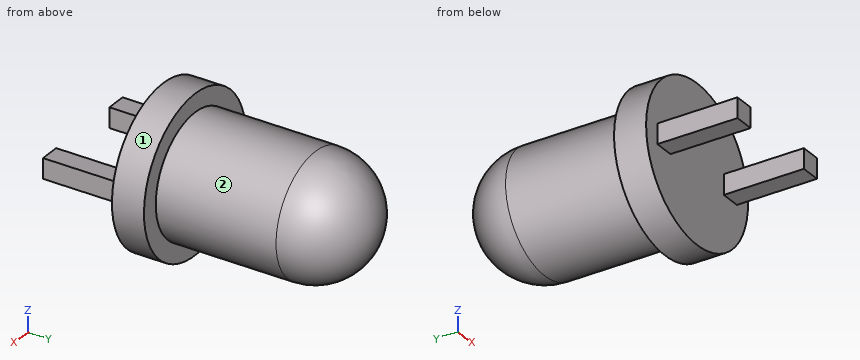
from build123d import *

# Parameters (mm, degrees)
SKETCH_1_W      = 1.95
SKETCH_1_H      = 0.8
SKETCH_2_W      = 0.5
SKETCH_2_H      = 0.5
EXTRUDE_1_DEPTH = 2


with BuildPart() as part:
    # Эскиз1 → Повернуть1 (revolve)
    with BuildSketch(Plane.XY, mode=Mode.PRIVATE) as revolve_1_sk:
        with BuildLine():
            Line((-1.5, 0.8), (0, 0.8))
            Line((0, 0.8), (0, 5.3))
            ThreePointArc((0, 5.3), (-1.060660172, 4.860660172), (-1.5, 3.8))
            Line((-1.5, 3.8), (-1.5, 0.8))
        make_face()
        with Locations((-0.975, 0.4)):
            Rectangle(SKETCH_1_W, SKETCH_1_H)
    revolve(revolve_1_sk.sketch.rotate(Axis((0, 8.783857323, 0), (0, -1, 0)), 270), axis=Axis((0, 8.783857323, 0), (0, -1, 0)))

    # Эскиз2 → Бобышка-Вытянуть1 (add)
    with BuildSketch(Plane.XZ):
        with Locations((-1.27, 0)):
            Rectangle(SKETCH_2_W, SKETCH_2_H)
        with Locations((1.27, 0)):
            Rectangle(SKETCH_2_W, SKETCH_2_H)
    extrude(amount=EXTRUDE_1_DEPTH)


solid = part.part
The model under review builds one solid part; all positions refer to its coordinate system, in mm. Face numbers are marked on the shaded views. A direction names the side the tool comes from. Coordinates: 2 decimals unless noted, no trailing zeros. Write each loop counter-clockwise with the first axis right and the second up, starting at its lowest first coordinate (ties: lowest second). Pieces come first, ordered by that corner, then holes. Notation, with made-up numbers: (14, -6.75) -> (31, -6.75) arc R14 cw to (31, 0.25) -> close; hole circle Ø2 at (47.25, 66). An arc over 180 degrees is marked (long way). Answer in a Markdown table with one row per item.
1. Wall thickness on probe 1 along X at (y, z) = (-0.5, -0.1); probe 2 along X at (y, z) = (4.5, 0.85); probe 3 along Y at (x, z) = (0.1, -1.7): over which ranges is each line inside the solid? List them lowest first. Write a range as [from, to].
Answers below:
| item | result |
|---|---|
| probe 1 | x = [-1.52, -1.02], [1.02, 1.52] |
| probe 2 | x = [-1.02, 1.02] |
| probe 3 | y = [0, 0.8] |
2. For the marked faces 1 and 2, list the 3-axis set-ups (+Z, -Z, +X, -X, +Y, -Y) from which the entire face can be reached by the end or side of a thin tool; tool diameter is ignored.
Answers below:
| item | result |
|---|---|
| face 1 | +Y, -Y |
| face 2 | +Y |
3. We need section D-D, the plane y = 1.5. State the section outline as (x, z) points, and give its area (3 significant figures).
Answers below:
| item | result |
|---|---|
| outline | circle Ø3 at (0, 0) |
| area | 7.07 mm^2 |
4. Clearance check with flat-ended pins moving along their axes: pin 1 Ø0.6 at (x, y) = (-1.5, -1) entering from -Z; pin 2 Ø0.6 at (y, z) = (-1, 0) entering from -X; pin 3 Ø0.6 at (x, y) = (1.5, -1) entering from +Z. State where each tip first meets the part, or that it passes through.
Answers below:
| item | result |
|---|---|
| pin 1 | stops at z = -0.25 |
| pin 2 | stops at x = -1.52 |
| pin 3 | stops at z = 0.25 |
5. We need section A-A, the plane y = -1. State the section outline as (x, z) points.
Answers below:
| item | result |
|---|---|
| outline | (-1.52, -0.25) -> (-1.02, -0.25) -> (-1.02, 0.25) -> (-1.52, 0.25) -> close; (1.02, -0.25) -> (1.52, -0.25) -> (1.52, 0.25) -> (1.02, 0.25) -> close |
6. We need section B-B, the plane x = 0. State the section outline as (y, z) points.
Answers below:
| item | result |
|---|---|
| outline | (0, -1.95) -> (0.8, -1.95) -> (0.8, -1.5) -> (3.8, -1.5) arc R1.5 ccw to (3.8, 1.5) -> (0.8, 1.5) -> (0.8, 1.95) -> (0, 1.95) -> close |
7. We need section C-C, the plane z = 0. State the section outline as (x, y) points.
Answers below:
| item | result |
|---|---|
| outline | (-1.95, 0) -> (-1.52, 0) -> (-1.52, -2) -> (-1.02, -2) -> (-1.02, 0) -> (1.02, 0) -> (1.02, -2) -> (1.52, -2) -> (1.52, 0) -> (1.95, 0) -> (1.95, 0.8) -> (1.5, 0.8) -> (1.5, 3.8) arc R1.5 ccw to (-1.5, 3.8) -> (-1.5, 0.8) -> (-1.95, 0.8) -> close |
